Read the model definition and answer for the solid it produces. Units are mm, in the model's axes. Face numbers are marked on the shaded views. A direction names the side the tool comes from. Coordinates: 2 decimals unless noted, no trailing zeros. Loops run counter-clockwise (first coordinate to the right, second up) from the corner with the lowest first, then second, coordinate; pieces in that order, holes last.
from build123d import *

# Parameters (mm, degrees)
REVOLVE1_ANGLE     = 180
FILLET1_R          = 3
SKETCH2_W          = 30
SKETCH2_H          = 0.5
SKETCH3_R          = 1.15
CUT_EXTRUDE1_DEPTH = 5


with BuildPart() as part:
    # Sketch1 → Revolve1 (revolve)
    with BuildSketch(Plane.XY):
        Polygon((0, 40), (-27.5, 40), (-22.5, 0), (-18.530888493, 0.496138938), (-22.968871126, 36), (-13, 36), (-13, 28.277027027), (-3, 28.277027027), (-3, 36), (0, 36), align=None)
    revolve(axis=Axis((0, 40, 0), (0, -1, 0)), revolution_arc=REVOLVE1_ANGLE)

    # Fillet1
    fillet1_edges = [part.edges().sort_by_distance(p)[0] for p in [
        (0, 40, -27.5),
    ]]
    fillet(fillet1_edges, radius=FILLET1_R)

    # Sketch2 → Cut-Revolve1 (revolve, cut)
    with BuildSketch(Plane.XY):
        with Locations((1, 32.75)):
            Rectangle(SKETCH2_W, SKETCH2_H)
    revolve(axis=Axis((-14, 32.5, 0), (1, 0, 0)), mode=Mode.SUBTRACT)

    # Sketch3 → Cut-Extrude1 (cut)
    with BuildSketch(Plane.XY):
        with Locations((-24.309743639, 30.602464611)):
            Circle(SKETCH3_R)
        with Locations((-21.033834323, 4.395190082)):
            Circle(SKETCH3_R)
        with Locations((21.033834323, 4.395190082)):
            Circle(SKETCH3_R)
        with Locations((24.309743639, 30.602464611)):
            Circle(SKETCH3_R)
    extrude(amount=-CUT_EXTRUDE1_DEPTH, mode=Mode.SUBTRACT)


solid = part.part
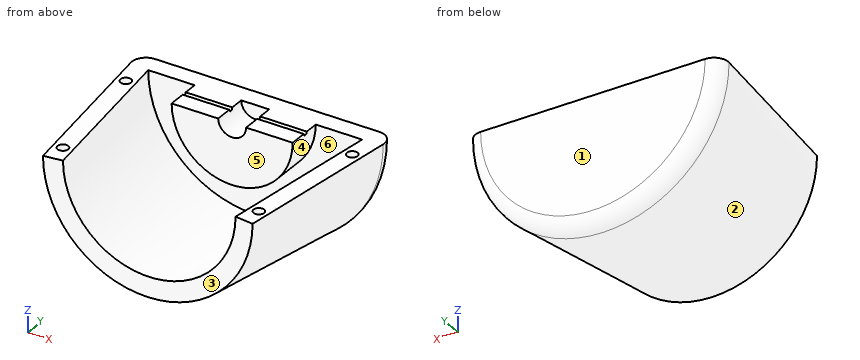
Item 1: Determine the mould class of the marked faces 1, 2 and 3 for opening direction X: released by +X, released by -X, zero draft, split by the parting line, or undercut.
Numbers:
face 1: zero draft
face 2: split by the parting line
face 3: undercut
Item 2: A cutting plane is placed at B-B on y = 23. Determine the outline of the cut face in (x, z) (3 decimals).
Numbers:
outline: (-25.375, 0) arc R25.375 ccw to (25.375, 0) - (21.344, 0) arc R21.344 cw to (-21.344, 0) - close
Item 3: A cutting plane is placed at A-A on x = 0. Determine the outline of the cut face in (y, z), then the cut area to 3 significant figures.
Numbers:
outline: (0, -22.5) - (36.63, -27.08) arc R3 ccw to (40, -24.1) - (40, 0) - (36, 0) - (36, -3) - (28.28, -3) - (28.28, -13) - (36, -13) - (36, -22.97) - (0.5, -18.53) - close
area: 328 mm2
Item 4: Which of the six approach directions +Z, -Z, +X, -X, +Y, -Y give full straight-line access (tool end or side, diameter ignored) to the marked faces 4, 5 and 6?
Numbers:
face 4: -Y
face 5: +Z, -Y
face 6: none
Item 5: Given pin 1 (6 mm diameter, centred on x = 20.5, y = 25.5, fed in from -Z); pin 2 (10 mm diameter, centred on y = 4, z = -7, fed in from +X); pin 3 (4 mm diameter, centred on x = 7, z = -7.5, fed in from -Y); pin 4 (3.5 mm diameter, centred on x = -21.03, y = 4.4, fed in from +Z), each flat-ended and moving along its own axis, determine where each tip first touches the part or whether it passes through.
Numbers:
pin 1: stops at z = -18.85
pin 2: stops at x = 23.19
pin 3: stops at y = 28.28
pin 4: stops at z = 0
Item 6: Find the intervals of material crossed by line 1 along X through (y, z) = (31.5, -6.75); line 2 along Y through (x, z) = (12.5, -12); line 3 along X through (y, z) = (35.5, -13.5), in increasing order.
Numbers:
line 1: x = -25.56 to -21.37, -11.11 to 11.11, 21.37 to 25.56
line 2: y = 36 to 40
line 3: x = -23.31 to -18.51, 18.51 to 23.31
